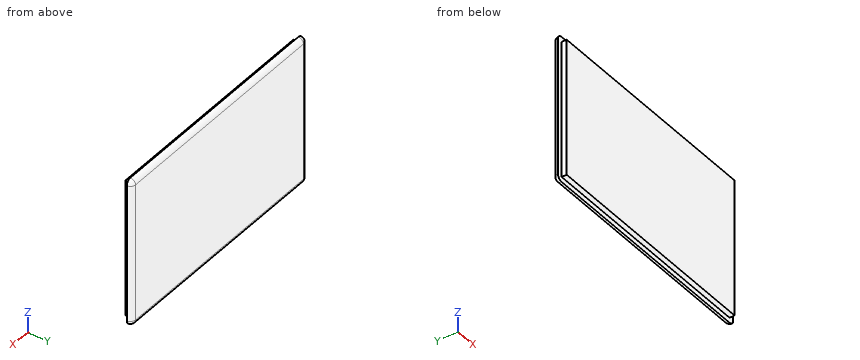
from build123d import *

# Parameters (mm, degrees)
SKETCH_1_W      = 46
SKETCH_1_H      = 27
EXTRUDE_1_DEPTH = 1
SKETCH_2_W      = 48
SKETCH_2_H      = 29
EXTRUDE_2_DEPTH = 1
FILLET_1_R      = 1


with BuildPart() as part:
    # ｽｹｯﾁ1 → ﾎﾞｽ - 押し出し1 (new body)
    with BuildSketch(Plane(origin=(0, 0, 0), x_dir=(1, 0, 0), z_dir=(0, 1, 0))):
        with Locations((-24.456990453, 23.251505547)):
            Rectangle(SKETCH_1_W, SKETCH_1_H)
    extrude(amount=EXTRUDE_1_DEPTH)

    # ｽｹｯﾁ2 → ﾎﾞｽ - 押し出し2 (add)
    with BuildSketch(Plane(origin=(0, 1, 0), x_dir=(1, 0, 0), z_dir=(0, 1, 0))):
        with Locations((-24.456990453, 23.251505547)):
            Rectangle(SKETCH_2_W, SKETCH_2_H)
    extrude(amount=EXTRUDE_2_DEPTH)

    # ﾌｨﾚｯﾄ1
    fillet_1_edges = [part.edges().sort_by_distance(p)[0] for p in [
        (-48.456990453, 1.5, -37.751505547),
        (-48.456990453, 1.5, -8.751505547),
        (-0.456990453, 1.5, -8.751505547),
        (-0.456990453, 1.5, -37.751505547),
        (-48.456990453, 2, -23.251505547),
        (-24.456990453, 2, -8.751505547),
        (-0.456990453, 2, -23.251505547),
        (-24.456990453, 2, -37.751505547),
    ]]
    fillet(fillet_1_edges, radius=FILLET_1_R - 0.0001)  # a hair under: the kernel refuses the full size


solid = part.part
Input: part model. Units: mm. Frame: model coordinates. Coordinates: 2 decimals unless noted, no trailing zeros. Loops run counter-clockwise (first coordinate to the right, second up) from the corner with the lowest first, then second, coordinate; pieces in that order, holes last. Notation, with made-up numbers: (-24.5, 18) -> (-14.5, 18) arc R21 cw to (-14.5, 39) -> close; hole circle Ø7 at (-20, 22.5). An arc over 180 degrees is marked (long way). Write item = value, one per line. Start each with the question number.
Item 1: First-contact query: P1, Ø0.8, axis at x = -33, y = 0.5, coming from the -Z side; P2, Ø0.5, axis at y = 0.5, z = -22.5, coming from the +X side; P3, Ø0.5, axis at x = -31, y = 0.5, coming from the +Z side. Flat tips, straight axial feed; report the tip coordinate or a pass-through.
Item 2: Cut plane C-C, the plane y = 0.3. Return loops of the section in (x, z), plus the area to 3 significant figures.
Item 3: Material intervals for line 1 (X direction, y = 1.05, z = -16.25); line 2 (Z direction, x = -13.5, y = 0.8); line 3 (X direction, y = 0.1, z = -35.75), sorted ascending.
Ans:
q1.P1 = -36.75
q1.P2 = -1.46
q1.P3 = -9.75
q2.outline = (-47.46, -36.75) -> (-1.46, -36.75) -> (-1.46, -9.75) -> (-47.46, -9.75) -> close
q2.area = 1,240 mm²
q3.line_1 = -48.46 to -0.46
q3.line_2 = -36.75 to -9.75
q3.line_3 = -47.46 to -1.46
